For this review, take the finished solid that the model builds, in its own axes (mm). A direction names the side the tool comes from. Round coordinates to 2 decimals unless told otherwise and drop trailing zeros. Order: outer loops, then holes, each group sorted by start corner. A loop starts at its lowest first (then second) coordinate and runs counter-clockwise, first axis right, second up. Notation, with made-up numbers: (-37, -23.5) - (21, -23.5) arc R19 cw to (21, -4.5) - close; hole circle Ø5 at (11, 8). An arc over 180 degrees is marked (long way). One line per question, with ' | ' between items.
```python
from build123d import *

# Parameters (mm, degrees)
SKETCH_1_R      = 2.55
SKETCH_1_W      = 55
SKETCH_1_H      = 20
EXTRUDE_1_DEPTH = 3


with BuildPart() as part:
    # 草图1 → 凸台-拉伸1 (new body)
    with BuildSketch(Plane(origin=(0, 0, 0), x_dir=(1, 0, 0), z_dir=(0, 1, 0))):
        with BuildLine():
            Line((16.20771131, 68.233643966), (16.20771131, 126.233643966))
            ThreePointArc((16.20771131, 126.233643966), (17.965070623, 130.476284653), (22.20771131, 132.233643966))
            Line((22.20771131, 132.233643966), (260.20771131, 132.233643966))
            ThreePointArc((260.20771131, 132.233643966), (264.450351998, 130.476284653), (266.20771131, 126.233643966))
            Line((266.20771131, 126.233643966), (266.20771131, 18.233643966))
            ThreePointArc((266.20771131, 18.233643966), (264.450351998, 13.991003279), (260.20771131, 12.233643966))
            Line((260.20771131, 12.233643966), (22.20771131, 12.233643966))
            ThreePointArc((22.20771131, 12.233643966), (17.965070623, 13.991003279), (16.20771131, 18.233643966))
            Line((16.20771131, 18.233643966), (16.20771131, 36.233643966))
            Line((16.20771131, 36.233643966), (26.20771131, 46.233643966))
            Line((26.20771131, 46.233643966), (48.20771131, 46.233643966))
            Line((48.20771131, 46.233643966), (48.20771131, 58.233643966))
            Line((48.20771131, 58.233643966), (26.20771131, 58.233643966))
            Line((26.20771131, 58.233643966), (16.20771131, 68.233643966))
        make_face()
        with Locations(Location((22.20771131, 126.233643966, 0), (0, 0, 270))):
            Circle(SKETCH_1_R, mode=Mode.SUBTRACT)
        with Locations(Location((260.20771131, 126.233643966, 0), (0, 0, 270))):
            Circle(SKETCH_1_R, mode=Mode.SUBTRACT)
        with Locations(Location((141.20771131, 122.233643966, 0), (0, 0, 270))):
            Circle(SKETCH_1_R, mode=Mode.SUBTRACT)
        with Locations(Location((22.20771131, 18.233643966, 0), (0, 0, 270))):
            Circle(SKETCH_1_R, mode=Mode.SUBTRACT)
        with Locations(Location((260.20771131, 18.233643966, 0), (0, 0, 270))):
            Circle(SKETCH_1_R, mode=Mode.SUBTRACT)
        with Locations(Location((141.20771131, 22.233643966, 0), (0, 0, 270))):
            Circle(SKETCH_1_R, mode=Mode.SUBTRACT)
        with Locations(Location((260.20771131, 72.233643966, 0), (0, 0, 270))):
            Circle(SKETCH_1_R, mode=Mode.SUBTRACT)
        with Locations(Location((22.20771131, 72.233643966, 0), (0, 0, 270))):
            Circle(SKETCH_1_R, mode=Mode.SUBTRACT)
        with Locations((136.20771131, 107.233643966)):
            Rectangle(SKETCH_1_W, SKETCH_1_H, mode=Mode.SUBTRACT)
    extrude(amount=EXTRUDE_1_DEPTH)


solid = part.part
```
(1) We need section C-C on z = -51. State the section outline as (x, y) points, plus the area to 3 significant figures.
Output values:
outline: (48.21, 0) - (266.21, 0) - (266.21, 3) - (48.21, 3) - close | area: 654 mm^2
(2) Insertion check: pin 1 (10 mm diameter, centred on x = 239.5, z = -54, fed in from -Y); pin 2 (4 mm diameter, centred on x = 141.21, z = -22.23, fed in from -Y). Each pin has a flat end and moves straight along its axis. Give the tip position at first contact, or say it passes through.
Output values:
pin 1: y = 0 | pin 2: through
(3) For probe 1 along X at (y, z) = (2.05, -108.5); probe 2 along Z at (x, y) = (41, 2.35); probe 3 along X at (y, z) = (2.6, -124.5), list the stretches that pass through material, from the lowest coordinate up. Write a range as [from, to].
Output values:
probe 1: [16.21, 108.71], [163.71, 266.21] | probe 2: [-132.23, -58.23], [-46.23, -12.23] | probe 3: [16.21, 20.34], [24.08, 140.04], [142.38, 258.34], [262.08, 266.21]
(4) We need section A-A on x = 154. State the section outline as (y, z) points, plus the area to 3 significant figures.
Output values:
outline: (0, -132.23) - (3, -132.23) - (3, -117.23) - (0, -117.23) - close; (0, -97.23) - (3, -97.23) - (3, -12.23) - (0, -12.23) - close | area: 300 mm^2
(5) We need section B-B on y = 1.55. Give the number of separate pieces and of enclosed holes in the cut face, plus the area to 3 significant figures.
Output values:
separate pieces: 1 | enclosed holes: 9 | area: 28,200 mm^2
(6) For faces 4 (the flat face through (21.138, 1.479, -41.164)), 5 (the cylindrical face through (262.736, 1.479, -126.566)), list the 3-axis set-ups (+Z, -Z, +X, -X, +Y, -Y) from which the entire face can be reached by the end or side of a thin tool; tool diameter is ignored.
Output values:
face 4: -X, +Y, -Y | face 5: +Y, -Y
(7) Mouldability with a two-part tool opening along Z and no side actions: class faces 1 (the cylindrical face through (20.66, 1.48, -20.26)), 2 (the cylindrical face through (264.403, 1.479, -130.523)), 3 (the cylindrical face through (264.5, 1.48, -14.04)) as released by +Z, released by -Z, zero draft, split by the parting line, or undercut.
Output values:
face 1: undercut | face 2: released by -Z | face 3: released by +Z
